CAD build for the part. Positions are in the model's coordinates, mm. A direction names the side the tool comes from. Round coordinates to 2 decimals unless told otherwise and drop trailing zeros. Order: outer loops, then holes, each group sorted by start corner. A loop starts at its lowest first (then second) coordinate and runs counter-clockwise, first axis right, second up. Notation, with made-up numbers: M 38.25,-40 L 89.25,-40 A35 cw 89.25,-5 Z; hole C -6.5,70 d10. An arc over 180 degrees is marked long. Put each result on its own line as item: value.
```python
from build123d import *

# Parameters (mm, degrees)
EXTRUDE_1_DEPTH     = 65
SHELL_1_T           = -4
CUT_EXTRUDE_1_REACH = 686.315
CUT_EXTRUDE_2_REACH = 686.315
FILLET_2_R          = 10
FILLET_3_R          = 7


with BuildPart() as part:
    # 草图1 → 凸台-拉伸1 (new, symmetric)
    with BuildSketch(Plane.XY):
        with BuildLine():
            Line((-58.512960007, 634.252160061), (-100.209989819, 31.352160061))
            ThreePointArc((-100.209989819, 31.352160061), (-30.672049595, 100.420243844), (65.590010181, 81.993600753))
            Line((65.590010181, 81.993600753), (25.187039993, 664.293600753))
            ThreePointArc((25.187039993, 664.293600753), (-6.261361418, 620.292452643), (-58.512960007, 634.252160061))
        make_face()
    extrude(amount=EXTRUDE_1_DEPTH, both=True)

    # 抽壳1
    shell_1_openings = [part.faces().sort_by_distance(p)[0] for p in [
        (-30.672049595, 100.420243844, 0),
        (-6.261361418, 620.292452643, 0),
    ]]
    offset(amount=SHELL_1_T, openings=shell_1_openings, kind=Kind.INTERSECTION)

    # 草图2 → 切除-拉伸1 (cut, up to next)
    with BuildSketch(Plane(origin=(70.93763316, 4.922017994, 0), x_dir=(0, 0, -1), z_dir=(0.9976015076237793, 0.06921872569444461, 0)), mode=Mode.PRIVATE) as cut_extrude_1_sk1:
        with BuildLine():
            Line((-40, 660.956882804), (-40, 600.956882804))
            ThreePointArc((-40, 600.956882804), (0, 560.956882804), (40, 600.956882804))
            Line((40, 600.956882804), (40, 660.956882804))
            Line((40, 660.956882804), (-40, 660.956882804))
        make_face()
    cut_extrude_1_tool1 = extrude(cut_extrude_1_sk1.sketch, amount=-CUT_EXTRUDE_1_REACH, mode=Mode.PRIVATE) & part.part
    add(cut_extrude_1_tool1.solids().sort_by_distance((28.381063, 618.26036, 0))[0], mode=Mode.SUBTRACT)

    # 草图3 → 切除-拉伸2 (cut, up to next)
    with BuildSketch(Plane(origin=(70.93763316, 4.922017994, 0), x_dir=(0, 0, -1), z_dir=(0.9976015076237793, 0.06921872569444461, 0)), mode=Mode.PRIVATE) as cut_extrude_2_sk1:
        with BuildLine():
            Line((-58.950365875, 77.256882804), (-44.505713851, 173.908306305))
            ThreePointArc((-44.505713851, 173.908306305), (-12.328164841, 210.535241733), (34.320074836, 196.362422882))
            Line((34.320074836, 196.362422882), (59.003367844, 167.256882804))
            Line((59.003367844, 167.256882804), (59.003367844, 77.256882804))
            Line((59.003367844, 77.256882804), (-58.950365875, 77.256882804))
        make_face()
    cut_extrude_2_tool1 = extrude(cut_extrude_2_sk1.sketch, amount=-CUT_EXTRUDE_2_REACH, mode=Mode.PRIVATE) & part.part
    add(cut_extrude_2_tool1.solids().sort_by_distance((61.423964, 142.035935, -3.018476))[0], mode=Mode.SUBTRACT)

    # 圆角2
    fillet_2_edges = [part.edges().sort_by_distance(p)[0] for p in [
        (45.388525087, 373.143600753, -65),
        (45.388525087, 373.143600753, 65),
        (-79.361474913, 332.802160061, 65),
        (-79.361474913, 332.802160061, -65),
    ]]
    fillet(fillet_2_edges, radius=FILLET_2_R)

    # 圆角3
    # the kernel refuses this fillet: 7 mm, written as the material it adds along each edge
    with BuildSketch(Plane(origin=(-53.567364395, 647.786430481, 61), x_dir=(0, 0, -1), z_dir=(-0.06899595830556898, -0.9976169393797883, 0))) as fillet_3_piece_1_section:
        with BuildLine():
            CenterArc((FILLET_3_R, FILLET_3_R), FILLET_3_R, 180, 90)
            Line((0, FILLET_3_R), (0, 0))
            Line((0, 0), (FILLET_3_R, 0))
        make_face()
    fillet_3_piece_1 = extrude(amount=622.701795047, mode=Mode.PRIVATE)
    fillet_3_piece_1 = fillet_3_piece_1 - Plane(origin=(-22.307707086, 665, 59.408269391), x_dir=(0.9998894121907572, -0.014871563092767819, 0), z_dir=(0, 0, 1)) * Cylinder(47.5, 1274, mode=Mode.PRIVATE)
    fillet_3_piece_1 = fillet_3_piece_1 - Plane(origin=(0, 0, 59.408269391), x_dir=(-0.9543808554191496, 0.29859200057840163, 0), z_dir=(0, 0, 1)) * Cylinder(105, 1274, mode=Mode.PRIVATE)
    add(fillet_3_piece_1)
    with BuildSketch(Plane(origin=(21.055790856, 666.046599906, -61), x_dir=(0, 0, 1), z_dir=(0.06921872569444461, -0.9976015076237793, 0))) as fillet_3_piece_2_section:
        with BuildLine():
            CenterArc((FILLET_3_R, FILLET_3_R), FILLET_3_R, 180, 90)
            Line((0, FILLET_3_R), (0, 0))
            Line((0, 0), (FILLET_3_R, 0))
        make_face()
    fillet_3_piece_2 = extrude(amount=599.735885548, mode=Mode.PRIVATE)
    fillet_3_piece_2 = fillet_3_piece_2 - Plane(origin=(-22.307707086, 665, -57.567140741), x_dir=(0.9998894121907572, -0.014871563092767819, 0), z_dir=(0, 0, 1)) * Cylinder(47.5, 1228, mode=Mode.PRIVATE)
    fillet_3_piece_2 = split(fillet_3_piece_2, bisect_by=Plane(origin=(45.190808802, 311.119705723, 59.715559847), z_dir=(-0.04476996432990456, 0.6452384591552827, -0.7626683296956915)), keep=Keep.TOP, mode=Mode.PRIVATE)
    fillet_3_piece_2 = split(fillet_3_piece_2, bisect_by=Plane(origin=(38.306109231, 410.34410782, -59.003367844), z_dir=(0, 0, 1)), keep=Keep.TOP, mode=Mode.PRIVATE)
    add(fillet_3_piece_2)
    with BuildSketch(Plane(origin=(21.055790856, 666.046599906, -61), x_dir=(0, 0, 1), z_dir=(0.06921872569444461, -0.9976015076237793, 0))) as fillet_3_piece_3_section:
        with BuildLine():
            CenterArc((FILLET_3_R, FILLET_3_R), FILLET_3_R, 180, 90)
            Line((0, FILLET_3_R), (0, 0))
            Line((0, 0), (FILLET_3_R, 0))
        make_face()
    fillet_3_piece_3 = extrude(amount=599.735885548, mode=Mode.PRIVATE)
    fillet_3_piece_3 = fillet_3_piece_3 - Plane(origin=(-22.307707086, 665, -60.275474349), x_dir=(0.9998894121907572, -0.014871563092767819, 0), z_dir=(0, 0, 1)) * Cylinder(47.5, 1228, mode=Mode.PRIVATE)
    fillet_3_piece_3 = split(fillet_3_piece_3, bisect_by=Plane(origin=(43.813424167, 307.914474781, 57.084700881), z_dir=(-0.04476996432990456, 0.6452384591552827, -0.7626683296956915)), keep=Keep.TOP, mode=Mode.PRIVATE)
    fillet_3_piece_3 = split(fillet_3_piece_3, bisect_by=Plane(origin=(36.9241767, 407.204422564, -59.003367844), z_dir=(0, 0, -1)), keep=Keep.TOP, mode=Mode.PRIVATE)
    add(fillet_3_piece_3)
    with BuildSketch(Plane(origin=(21.055790856, 666.046599906, -61), x_dir=(0, 0, 1), z_dir=(0.06921872569444461, -0.9976015076237793, 0))) as fillet_3_piece_4_section:
        with BuildLine():
            CenterArc((FILLET_3_R, FILLET_3_R), FILLET_3_R, 180, 90)
            Line((0, FILLET_3_R), (0, 0))
            Line((0, 0), (FILLET_3_R, 0))
        make_face()
    fillet_3_piece_4 = extrude(amount=599.735885548, mode=Mode.PRIVATE)
    fillet_3_piece_4 = split(fillet_3_piece_4, bisect_by=Plane(origin=(55.090839822, 145.685566131, -80.827437921), z_dir=(0.04476996432990456, -0.6452384591552827, 0.7626683296956915)), keep=Keep.TOP, mode=Mode.PRIVATE)
    fillet_3_piece_4 = fillet_3_piece_4 - Plane(origin=(0, 0, -60.266827154), x_dir=(-0.9543808554191496, 0.29859200057840163, 0), z_dir=(0, 0, 1)) * Cylinder(105, 1228, mode=Mode.PRIVATE)
    fillet_3_piece_4 = split(fillet_3_piece_4, bisect_by=Plane(origin=(56.29778362, 128.290721879, -59.003367844), z_dir=(0, 0, -1)), keep=Keep.TOP, mode=Mode.PRIVATE)
    add(fillet_3_piece_4)
    with BuildSketch(Plane(origin=(-96.531271483, 26.56857156, -61), x_dir=(0.9976169393797882, -0.06899595830556898, 0), z_dir=(0.06899595830556898, 0.9976169393797883, 0))) as fillet_3_piece_5_section:
        with BuildLine():
            CenterArc((FILLET_3_R, -FILLET_3_R), FILLET_3_R, 90, 90)
            Line((0, -FILLET_3_R), (0, 0))
            Line((0, 0), (FILLET_3_R, 0))
        make_face()
    fillet_3_piece_5 = extrude(amount=622.701795047, mode=Mode.PRIVATE)
    fillet_3_piece_5 = fillet_3_piece_5 - Plane(origin=(-22.307707086, 665, -59.408268286), x_dir=(0.9998894121907572, -0.014871563092767819, 0), z_dir=(0, 0, 1)) * Cylinder(47.5, 1274, mode=Mode.PRIVATE)
    fillet_3_piece_5 = fillet_3_piece_5 - Plane(origin=(0, 0, -59.408268286), x_dir=(-0.9543808554191496, 0.29859200057840163, 0), z_dir=(0, 0, 1)) * Cylinder(105, 1274, mode=Mode.PRIVATE)
    add(fillet_3_piece_5)
    with BuildSketch(Plane(origin=(21.055790856, 666.046599906, 61), x_dir=(0, 0, -1), z_dir=(0.06921872569444461, -0.9976015076237793, 0))) as fillet_3_piece_6_section:
        with BuildLine():
            CenterArc((FILLET_3_R, -FILLET_3_R), FILLET_3_R, 90, 90)
            Line((0, -FILLET_3_R), (0, 0))
            Line((0, 0), (FILLET_3_R, 0))
        make_face()
    fillet_3_piece_6 = extrude(amount=599.735885548, mode=Mode.PRIVATE)
    fillet_3_piece_6 = fillet_3_piece_6 - Plane(origin=(-22.307707086, 665, 59.420291377), x_dir=(0.9998894121907572, -0.014871563092767819, 0), z_dir=(0, 0, 1)) * Cylinder(47.5, 1228, mode=Mode.PRIVATE)
    fillet_3_piece_6 = split(fillet_3_piece_6, bisect_by=Plane(origin=(40.666871165, 360.585918915, 17.156503264), z_dir=(-0.010231179084037917, 0.1474548913838828, 0.9890158633619169)), keep=Keep.TOP, mode=Mode.PRIVATE)
    fillet_3_piece_6 = fillet_3_piece_6 - Plane(origin=(0, 0, 59.420291377), x_dir=(-0.9543808554191496, 0.29859200057840163, 0), z_dir=(0, 0, 1)) * Cylinder(105, 1228, mode=Mode.PRIVATE)
    add(fillet_3_piece_6)


solid = part.part
```
Item 1: Mould opens along X. For faces 1 (the flat face through (59, 128, -59.003)), 2 (the flat face through (-74.765, 341.282, 0.756)), 3 (the cylindrical face through (-96.084, 42.343, 0.303)), 4 (the cylindrical face through (54.411, 214.613, 13.02)) say: pulls with the +X half, pulls with the -X half, needs draft (parallel to the pull), parting line crosses it, or undercut.
Answers below:
face 1: needs draft
face 2: undercut
face 3: undercut
face 4: pulls with the +X half
Item 2: Pin check, flat tips, straight feed: P1, Ø4, axis at y = 185, z = 22.5, coming from the +X side; P2, Ø8, axis at x = 26, y = 633.5, coming from the +Z side; P3, Ø3, axis at y = 512.5, z = 45.5, coming from the +X side; P4, Ø5, axis at x = 25.5, z = -8, coming from the +Y side. Stop position of each tip, or through.
Answers below:
P1: x = -85.44
P2: z = 63.84
P3: x = 35.82
P4: through
Item 3: Band-saw the part on B-B on x = -5.5. Give the cut face in (y, z), and give its area (3 significant figures).
Answers below:
outline: M 104.86,-65 L 620.57,-65 L 620.57,-61 L 104.86,-61 Z; M 104.86,61 L 620.57,61 L 620.57,65 L 104.86,65 Z
area: 4,130 mm²
Item 4: Tool access for faces 5 (the cylindrical face through (-76.8, 328.4, 62)), 6 (the flat face through (-18, 352, 61)): list every direction of +Z, -Z, +X, -X, +Y, -Y with a clear straight run to the whole face (end or side of a thin tool).
Answers below:
face 5: +Z, -X, +Y
face 6: -Y
Item 5: Band-saw the part on A-A on z = -12.5. Give the cut face in (x, y), and give its area (3 significant figures).
Answers below:
outline: M -100.21,31.35 A105 cw -95.32,44.03 L -54.77,630.33 A47.5 cw -58.51,634.25 Z; M 27.98,566.26 L 52.38,214.63 L 56.37,214.9 L 31.97,566.53 Z
area: 3,790 mm²
Item 6: Probe line 1 along Z through (x, y) = (-51, 567); line 2 along Z through (x, y) = (57, 131); line 3 along X through (y, z) = (420, 56). List the from-to ranges inside material, lowest first. Write a range as [from, to].
Answers below:
line 1: [-65, -61], [61, 65]
line 2: [-63.76, -59], [57.89, 63.76]
line 3: [-73.28, -69.03], [37.84, 42.09]
